```python
from build123d import *

# Parameters (mm, degrees)
BOSS_EXTRU_1_DEPTH = 20
ESQUISSE2_W        = 20
ESQUISSE2_H        = 30
BOSS_EXTRU_2_DEPTH = 20
ESQUISSE3_R        = 15
BOSS_EXTRU_3_DEPTH = 10


with BuildPart() as part:
    # Esquisse1 → Boss.-Extru.1 (new body)
    with BuildSketch(Plane.XY):
        Polygon((110, 0), (-110, 0), (-110, 40), (-90, 40), (-90, 20), (-10, 20), (-10, 40), (10, 40), (10, 20), (90, 20), (90, 40), (110, 40), align=None)
    extrude(amount=BOSS_EXTRU_1_DEPTH)

    # Esquisse2 → Boss.-Extru.2 (add)
    with BuildSketch(Plane.XY.offset(20)):
        with Locations((0, -15)):
            Rectangle(ESQUISSE2_W, ESQUISSE2_H)
    extrude(amount=-BOSS_EXTRU_2_DEPTH)

    # Esquisse3 → Boss.-Extru.3 (add)
    with BuildSketch(Plane(origin=(0, 40, 0), x_dir=(1, 0, 0), z_dir=(0, 1, 0))):
        with Locations(Location((0, -10, 0), (0, 0, 270))):
            Circle(ESQUISSE3_R)
        with Locations(Location((-100, -10, 0), (0, 0, 270))):
            Circle(ESQUISSE3_R)
        with Locations(Location((100, -10, 0), (0, 0, 270))):
            Circle(ESQUISSE3_R)
    extrude(amount=BOSS_EXTRU_3_DEPTH)


solid = part.part
```
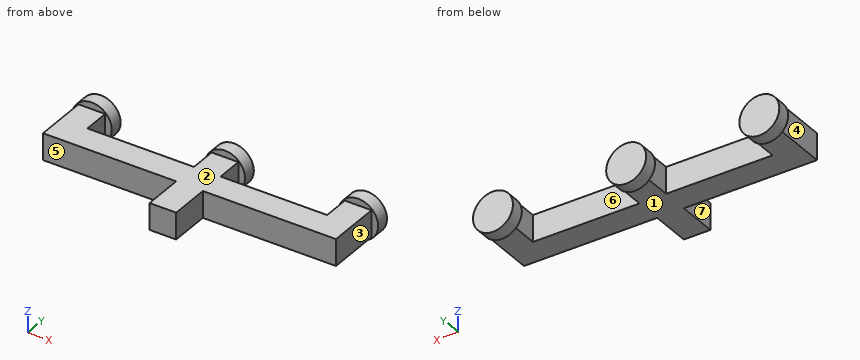
Source: CAD feature listing. Evaluate the final solid. Frame: model axes, mm. Face numbers are marked on the shaded views. A direction names the side the tool comes from. Give positions to 0.01 mm unless a question says otherwise; leave off trailing zeros. Loops run counter-clockwise (first coordinate to the right, second up) from the corner with the lowest first, then second, coordinate; pieces in that order, holes last. Notation, with made-up numbers: (3.25, 50.25) - (16.25, 50.25) arc R19 ccw to (16.25, 56.25) - close; hole circle Ø10 at (-3.5, 56.25). An arc over 180 degrees is marked (long way). Use CSV: the item, a comma, the result in double quotes. Start each with the question number.
1. Reachability of the marked faces 1, 2, 3 and 4 from +Z, -Z, +X, -X, +Y, -Y: full face, straight path, thin tool, end or side. Return the list, or none.
2. Section B-B (y = 34). Output: boundary loops of the cut face in (x, z).
3. Draft query along X for the marked faces 5, 6 and 7. Return one class per face: +X half, -X half, draft (parallel to the pull), parting line (faces both ways), or undercut.
4. Section D-D (y = -8.5). Output: boundary loops of the cut face in (x, z).
5. Section A-A (x = -100). Output: boundary loops of the cut face in (y, z), then the cut area to 3 significant figures.
6. Ray query, L1, parallel to X at y = 32, z = 14; L2, parallel to Z at x = 67, y = 11; L3, parallel to Y at x = -98, z = 21.5. Return the intervals inside material, ascending.
7. Pin query (flat end, axial travel): pin 1 (10 mm diameter, centred on x = 42.5, z = 9, fed in from -Y); pin 2 (10 mm diameter, centred on y = -21.5, z = 13, fed in from -X); pin 3 (8 mm diameter, centred on y = -0.5, z = 7, fed in from +X). Return the tip coordinate at first contact, or that it passes through.
8. Section C-C (z = 10). Output: boundary loops of the cut face in (x, y), then the cut area to 3 significant figures.
Response:
1,face 1,"-Z, +X, -X, -Y"
1,face 2,"+Z, +X, -X, -Y"
1,face 3,"+Z, -Z, +X, -Y"
1,face 4,"+Z, -Z, -X, -Y"
2,outline,"(-110, 0) - (-90, 0) - (-90, 20) - (-110, 20) - close; (-10, 0) - (10, 0) - (10, 20) - (-10, 20) - close; (90, 0) - (110, 0) - (110, 20) - (90, 20) - close"
3,face 5,"draft"
3,face 6,"undercut"
3,face 7,"-X half"
4,outline,"(-10, 0) - (10, 0) - (10, 20) - (-10, 20) - close"
5,outline,"(0, 0) - (40, 0) - (40, -5) - (50, -5) - (50, 25) - (40, 25) - (40, 20) - (0, 20) - close"
5,area,"1,100 mm²"
6,L1,"-110 to -90, -10 to 10, 90 to 110"
6,L2,"0 to 20"
6,L3,"40 to 50"
7,pin 1,"y = 0"
7,pin 2,"x = -10"
7,pin 3,"x = 110"
8,outline,"(-115, 40) - (-110, 40) - (-110, 0) - (-10, 0) - (-10, -30) - (10, -30) - (10, 0) - (110, 0) - (110, 40) - (115, 40) - (115, 50) - (85, 50) - (85, 40) - (90, 40) - (90, 20) - (10, 20) - (10, 40) - (15, 40) - (15, 50) - (-15, 50) - (-15, 40) - (-10, 40) - (-10, 20) - (-90, 20) - (-90, 40) - (-85, 40) - (-85, 50) - (-115, 50) - close"
8,area,"7,100 mm²"
